Here's how the part is built. I have some questions about the finished solid (model axes, mm). A direction names the side the tool comes from. Coordinates: 2 decimals unless noted, no trailing zeros. Loops run counter-clockwise (first coordinate to the right, second up) from the corner with the lowest first, then second, coordinate; pieces in that order, holes last. Notation, with made-up numbers: M -1.5,58 L 29.5,58 A9 cw 29.5,67 Z; hole C 66,-10 d9. An arc over 180 degrees is marked long. Use one line per item in the form item = value. Start each with the question number.
(1) Thinking about a two-plate mould opening in X: for faces 6 (the flat face through (66, 0, 10)), 7 (the cylindrical face through (56.624, -17.255, 4.83)), 8 (the flat face through (67, 30, 9)), 9 (the cylindrical face through (6.4, 19.86, 10.45)), which applies, +X half, -X half, draft (parallel to the pull), parting line (faces both ways), or undercut?
(2) Imagine slicing it at B-B, the plane y = 15. Please give me the cut outline in (x, z).
(3) Please list where these lines run through material, in increasing order: L1, parallel to Z at x = 66, y = -22; L2, parallel to Z at x = 70, y = -31; L3, parallel to Y at x = 104, z = 17.
(4) On a 3-axis mill with a long thin cutter (end or side, diameter ignored), from which of +Z, -Z, +X, -X, +Y, -Y can I reach the whole of each face in a straight line? I mean faces 1 (the cylindrical face through (86.83, -19.79, 12.52)), 2 (the flat face through (97.28, 20, 49)), 3 (the flat face through (97.28, 20, -29)), 4 (the flat face through (35.132, 20, 49)), 5 (the flat face through (35.132, 20, -29)). Say none if no direction works.
(5) Imagine slicing it at A-A, the plane z = 44. Please give me the cut outline in (x, y), and give its area (3 significant figures).
(6) Imagine slicing it at C-C, the plane y = -29. Please give me the cut outline in (x, z).
(7) Will these pins go through, and if not, where does the flat tip stop? P1, Ø17.5, axis at x = 66.21, z = 9.81, coming from the -Y side; P2, Ø16, axis at y = 17, z = -33, coming from the +X side; P3, Ø1, axis at x = 80.5, y = -25, coming from the +Z side.
```python
from build123d import *

# Parameters (mm, degrees)
SALIENTE_EXTRUIR1_DEPTH = 30
CROQUIS3_R              = 20.8
CROQUIS3_R_2            = 10.8
SALIENTE_EXTRUIR2_DEPTH = 35
REDONDEO1_R             = 5
REDONDEO4_R             = 10


with BuildPart() as part:
    # Croquis2 → Saliente-Extruir1 (new body)
    with BuildSketch(Plane(origin=(0, 0, 0), x_dir=(1, 0, 0), z_dir=(0, 1, 0))):
        with BuildLine():
            Line((35.131604566, 18.926463751), (35.131604566, 39.218716838))
            ThreePointArc((35.131604566, 39.218716838), (66.20576122, 70.292873492), (97.279917874, 39.218716838))
            Line((97.279917874, 39.218716838), (97.279917874, 18.926463751))
            ThreePointArc((97.279917874, 18.926463751), (126.019675086, -9.813293461), (97.279917874, -38.553050674))
            Line((97.279917874, -38.553050674), (97.279917874, -58.84530376))
            ThreePointArc((97.279917874, -58.84530376), (66.20576122, -89.919460414), (35.131604566, -58.84530376))
            Line((35.131604566, -58.84530376), (35.131604566, -38.553050674))
            ThreePointArc((35.131604566, -38.553050674), (6.391847353, -9.813293461), (35.131604566, 18.926463751))
        make_face()
    extrude(amount=SALIENTE_EXTRUIR1_DEPTH)

    # Croquis3 → Saliente-Extruir2 (add)
    with BuildSketch(Plane.XZ):
        with Locations(Location((66.20576122, 9.813293461, 0), (0, 0, 270))):
            Circle(CROQUIS3_R)
        with Locations(Location((66.20576122, 9.813293461, 0), (0, 0, 270))):
            Circle(CROQUIS3_R_2, mode=Mode.SUBTRACT)
    extrude(amount=SALIENTE_EXTRUIR2_DEPTH)

    # Redondeo1
    redondeo1_edges = [part.edges().sort_by_distance(p)[0] for p in [
        (66.20576122, 0, 30.613293461),
    ]]
    fillet(redondeo1_edges, radius=REDONDEO1_R)

    # Redondeo4
    redondeo4_edges = [part.edges().sort_by_distance(p)[0] for p in [
        (35.131604566, 0, 48.699177217),
        (6.391847353, 0, 9.813293461),
        (35.131604566, 0, -29.072590294),
        (66.20576122, 0, -70.292873492),
        (97.279917874, 0, -29.072590294),
        (126.019675086, 0, 9.813293461),
        (97.279917874, 0, 48.699177217),
        (66.20576122, 0, 89.919460414),
    ]]
    fillet(redondeo4_edges, radius=REDONDEO4_R)


solid = part.part
```
Answer:
q1.face_6 = undercut
q1.face_7 = undercut
q1.face_8 = draft
q1.face_9 = -X half
q2.outline = M 35.13,-39.22 A31.07 ccw 97.28,-39.22 L 97.28,-18.93 A28.74 ccw 97.28,38.55 L 97.28,58.85 A31.07 ccw 35.13,58.85 L 35.13,38.55 A28.74 ccw 35.13,-18.93 Z
q3.L1 = -10.99 to -0.98, 20.61 to 30.61
q3.L2 = -10.64 to -0.3, 19.92 to 30.26
q3.L3 = 0 to 30
q4.face_1 = -Y
q4.face_2 = +Z, +X, +Y, -Y
q4.face_3 = -Z, +X, +Y, -Y
q4.face_4 = +Z, -X, +Y, -Y
q4.face_5 = -Z, -X, +Y, -Y
q5.outline = M 35.13,10 A10 ccw 45.13,0 L 87.28,0 A10 ccw 97.28,10 L 97.28,30 L 35.13,30 Z
q5.area = 1,820 mm²
q6.outline = C 66.21,9.81 d41.6; hole C 66.21,9.81 d21.6
q7.P1 = 0
q7.P2 = 97.28
q7.P3 = 25.38
